Build history of the part. All positions in model axes, mm. Face numbers are marked on the shaded views. A direction names the side the tool comes from. Give positions to 0.01 mm unless a question says otherwise; leave off trailing zeros. Write each loop counter-clockwise with the first axis right and the second up, starting at its lowest first coordinate (ties: lowest second). Pieces come first, ordered by that corner, then holes. Notation, with made-up numbers: M 43.25,1.25 L 78.25,1.25 A20 cw 78.25,19.25 Z; hole C 73,36 d4. An arc over 180 degrees is marked long. Return JSON: item names as keys, results as strings. Group by question number.
Q1. Band-saw the part on D-D, the plane x = 17. Give the cut face in (y, z), then the cut area to 3 significant figures.
Q2. Tool access for the marked faces 4 and 5: list every direction of +Z, -Z, +X, -X, +Y, -Y with a clear straight run to the whole face (end or side of a thin tool).
Q3. Wall check: probe 1 along Y at (x, z) = (6, 5); probe 2 along Y at (x, z) = (-7, 4.25); probe 3 along X at (y, z) = (9, 4.5). Give the ranges that are in metal, low to high.
Q4. Pull direction X, two halves, no side cores. Call the marked faces 1, 2 and 3: +X half, -X half, draft (parallel to the pull), parting line (faces both ways), or undercut.
Q5. Flat gauge pins, fed straight in: pin 1 Ø12 at (x, y) = (0, -9.5) entering from -Z; pin 2 Ø5 at (y, z) = (5.5, 5.5) entering from +X; pin 3 Ø3 at (y, z) = (8.5, 5.5) entering from +X; pin 4 Ø4 at (x, z) = (-6.5, 5) entering from -Y. Where does each tip first touch, or does it go through?
Q6. Band-saw the part on B-B, the plane x = 6. Give the cut face in (y, z), then the cut area to 3 significant figures.
Q7. Band-saw the part on A-A, the plane z = 7.5. Give the cut face in (x, y), then the cut area to 3 significant figures.
Q8. Band-saw the part on C-C, the plane y = -7. Give the cut face in (x, z), then the cut area to 3 significant figures.
from build123d import *

# Parameters (mm, degrees)
BOSS_EXTRUDE1_DEPTH = 10


with BuildPart() as part:
    # Sketch1 → Boss-Extrude1 (new body)
    with BuildSketch(Plane.XY):
        with BuildLine():
            Line((-23, 0), (-23, 15))
            ThreePointArc((-23, 15), (-6.351498428, 37.105620727), (19.492040672, 27.209027416))
            ThreePointArc((19.492040672, 27.209027416), (19.044286348, 23.468920949), (15.294171401, 23.114635465))
            ThreePointArc((15.294171401, 23.114635465), (13.010187777, 24.473109029), (10.606601718, 25.606601718))
            ThreePointArc((10.606601718, 25.606601718), (-5.740251485, 28.858192988), (-15, 15))
            Line((-15, 15), (-15, 0))
            ThreePointArc((-15, 0), (10.606601718, -10.606601718), (0, 15))
            ThreePointArc((0, 15), (-3.535533906, 13.535533906), (-5, 10))
            Line((-5, 10), (-5, 0))
            Line((-5, 0), (-10, 0))
            Line((-10, 0), (-10, 11.180339887))
            Line((-10, 11.180339887), (-10, 14.866068747))
            ThreePointArc((-10, 14.866068747), (-8.022181222, 20.132313456), (-3.066666667, 22.794638746))
            ThreePointArc((-3.066666667, 22.794638746), (17.313771012, -15.140453538), (-23, 0))
        make_face()
    extrude(amount=BOSS_EXTRUDE1_DEPTH)


solid = part.part
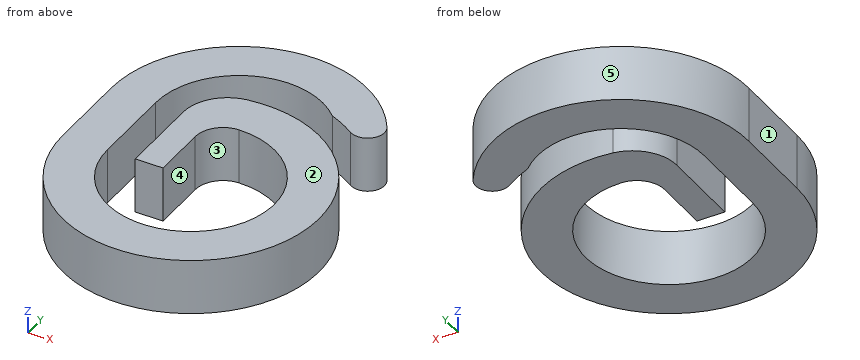
From the geometry:
{
 "1": {"outline": "M -15.49,0 L 15.49,0 L 15.49,10 L -15.49,10 Z; M 22.62,0 L 30.49,0 L 30.49,10 L 22.62,10 Z", "area": "389 mm^2"},
 "2": {"face 4": "+Z, -Z", "face 5": "+Z, -Z, +Y"},
 "3": {"probe 1": "y = -22.2 to -13.75, 13.75 to 22.2, 28.75 to 37.2", "probe 2": "y = -21.91 to -13.27, 0 to 21.11, 28.27 to 36.91", "probe 3": "x = -23 to -15, -10 to -5, 12 to 21.17"},
 "4": {"face 1": "-X half", "face 2": "draft", "face 3": "undercut"},
 "5": {"pin 1": "stops at z = 0", "pin 2": "stops at x = 22.8", "pin 3": "stops at x = 21.91", "pin 4": "stops at y = -22.56"},
 "6": {"outline": "M -22.2,0 L -13.75,0 L -13.75,10 L -22.2,10 Z; M 13.75,0 L 22.2,0 L 22.2,10 L 13.75,10 Z; M 28.75,0 L 37.2,0 L 37.2,10 L 28.75,10 Z", "area": "254 mm^2"},
 "7": {"outline": "M -23,0 A23 ccw long -3.07,22.79 A8 ccw -10,14.87 L -10,0 L -5,0 L -5,10 A5 cw 0,15 A15 cw long -15,0 L -15,15 A15 cw 10.61,25.61 A27.72 cw 15.29,23.11 A3 ccw 19.49,27.21 A23 ccw -23,15 Z", "area": "1,390 mm^2"},
 "8": {"outline": "M -21.91,0 L -13.27,0 L -13.27,10 L -21.91,10 Z; M 13.27,0 L 21.91,0 L 21.91,10 L 13.27,10 Z", "area": "173 mm^2"}
}
